The listing builds one solid part. Answer for the finished solid, in the listing's coordinates (mm). Round coordinates to 2 decimals unless told otherwise and drop trailing zeros. Use a Markdown table: item, result. Add a question column.
1) Each of these flat-tipped pins is pushed along its axis until it touches: P1, Ø5.5, axis at x = -119.11, z = 68.77, coming from the +Y side; P2, Ø8.5, axis at x = -78.74, z = -136.38, coming from the -Y side; P3, Ø5.5, axis at x = 119.11, z = 68.77, coming from the -Y side; P4, Ø6, axis at x = -157.48, z = 0, coming from the +Y side. Where does it stop, or does it pass through?
2) A cutting plane is placed at B-B (y = 5.25). State how many separate pieces and enclosed holes the cut face has, then the cut area to 3 significant figures.
3) Find the intervals of material crossed by probe 1 along X at (y, z) = (6.5, 0); probe 2 along Z at (x, y) = (0, 10.8); probe 3 along X at (y, z) = (1.5, -2), in increasing order. Write a range as from..to.
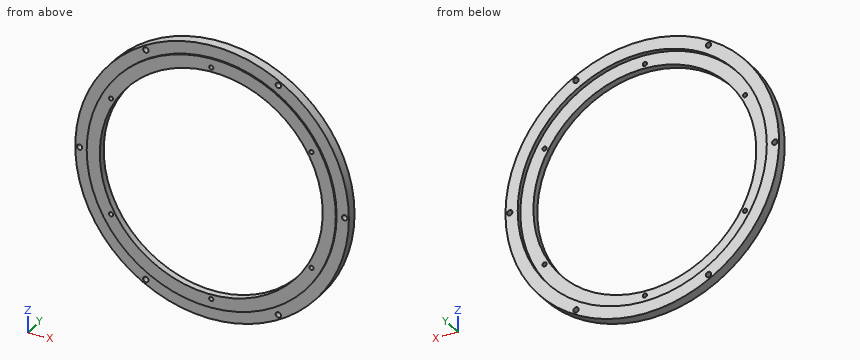
Autodesk Inventor part; units mm, degrees
ref_plane "YZ Plane" through (0, 0, 0) normal (1, 0, 0) x (0, 1, 0)
ref_plane "XZ Plane" through (0, 0, 0) normal (0, 1, 0) x (-1, 0, 0)
ref_plane "XY Plane" through (0, 0, 0) normal (0, 0, 1) x (1, 0, 0)
sketch "Sketch1" plane through (0, 0, 0) normal (0, 1, 0) x (-1, 0, 0)
  circle A0 centre (0, 0) radius 162.56 construction
  circle A1 centre (0, 0) radius 148.0058
  circle A2 centre (0, 0) radius 132.461
  dimension "d0" = 325.12
  dimension "d1" = 296.0116
  dimension "d2" = 264.922
extrude "Extrusion1" add sketch "Sketch1" along normal blind 1.778
sketch "Sketch2" plane through (0, 1.778, 0) normal (0, 1, 0) x (1, 0, 0)
  circle A0 centre (0, 0) radius 132.461
  circle A1 centre (0, 0) radius 162.56
  dimension "d5" = 325.12
extrude "Extrusion2" add sketch "Sketch2" along normal blind 12.192
sketch "Sketch3" plane through (0, 13.97, 0) normal (0, 1, 0) x (1, 0, 0)
  circle A0 centre (0, 0) radius 148.0058
  circle A1 centre (0, 0) radius 132.461
extrude "Extrusion3" cut sketch "Sketch3" against normal blind 5.588
sketch "Sketch4" plane through (0, 13.97, 0) normal (0, 1, 0) x (1, 0, 0)
  circle A0 centre (0, 0) radius 157.48 construction
  circle A1 centre (-157.48, 0) radius 3.9687
  circle A2 centre (-78.74, -136.3817) radius 3.9687
  circle A3 centre (78.74, -136.3817) radius 3.9687
  circle A4 centre (157.48, 0) radius 3.9687
  circle A5 centre (78.74, 136.3817) radius 3.9687
  circle A6 centre (-78.74, 136.3817) radius 3.9687
  dimension "d10" = 314.96
  dimension "d11" = 7.9375
  dimension "d14" = 360
hole "Hole1" at (-157.48, 13.97, 0) at (78.74, 13.97, -136.3817) at (-78.74, 13.97, -136.3817) at (157.48, 13.97, 0) at (78.74, 13.97, 136.3817) at (-78.74, 13.97, 136.3817) direction (0, -1, 0) diameter 6.4008 depth 22.9362
sketch "Sketch5" plane through (0, 8.382, 0) normal (0, 1, 0) x (1, 0, 0)
  line L0 (0, 0) -> (-122.3635, 70.6466) construction
  line L1 (0, 0) -> (141.2932, 0) construction
  line L2 (-122.3635, 70.6466) -> (0, 0) construction
  line L3 (0, 0) -> (-128.1768, -74.0029) construction
  circle A0 centre (0, 0) radius 148.0058 construction
  line L4 (0, 0) -> (148.0058, 0) construction
  circle A1 centre (0, 0) radius 137.541 construction
  circle A2 centre (-119.114, -68.7705) radius 3.175
  circle A3 centre (0, -137.541) radius 3.175
  circle A4 centre (119.114, -68.7705) radius 3.175
  circle A5 centre (119.114, 68.7705) radius 3.175
  circle A6 centre (0, 137.541) radius 3.175
  circle A7 centre (-119.114, 68.7705) radius 3.175
  dimension "d25" = 275.082
  dimension "d23" = 150
  dimension "d24" = 150
  dimension "d26" = 6.35
  dimension "d29" = 360
hole "Hole2" at (0, 8.382, 137.541) at (119.114, 8.382, 68.7705) at (119.114, 8.382, -68.7705) at (0, 8.382, -137.541) at (-119.114, 8.382, -68.7705) at (-119.114, 8.382, 68.7705) direction (0, -1, 0) diameter 4.9784 depth 19.05
properties part number "Turntable_2"
Entries:
| question | item | result |
|---|---|---|
| 1 | P1 | stops at y = 8.38 |
| 1 | P2 | stops at y = 1.78 |
| 1 | P3 | stops at y = 0 |
| 1 | P4 | passes through |
| 2 | separate pieces | 1 |
| 2 | enclosed holes | 13 |
| 2 | area | 27,600 mm² |
| 3 | probe 1 | x = -162.56..-160.68, -154.28..-132.46, 132.46..154.28, 160.68..162.56 |
| 3 | probe 2 | z = -162.56..-148.01, 148.01..162.56 |
| 3 | probe 3 | x = -147.99..-132.45, 132.45..147.99 |
